Verification items for the finished model (mm, model axes). A direction names the side the tool comes from. Round coordinates to 2 decimals unless told otherwise and drop trailing zeros. Write each loop counter-clockwise with the first axis right and the second up, starting at its lowest first coordinate (ties: lowest second). Pieces come first, ordered by that corner, then holes. Notation, with made-up numbers: (85, 5) - (89, 5) arc R6 ccw to (89, 13) - close; hole circle Ø6 at (11, 30). An arc over 180 degrees is marked (long way). Write each question's results on one line, items separated by ' | '.
```python
from build123d import *

# Parameters (mm, degrees)
SKETCH1_R           = 18.5
BOSS_EXTRUDE1_DEPTH = 6
SKETCH3_R           = 2
CUT_EXTRUDE1_DEPTH  = 6
SKETCH7_R           = 3
BOSS_EXTRUDE4_DEPTH = 18
FILLET3_R           = 8
SKETCH8_R           = 4.5
CUT_EXTRUDE2_DEPTH  = 10


with BuildPart() as part:
    # Sketch1 → Boss-Extrude1 (new body)
    with BuildSketch(Plane.XY):
        Circle(SKETCH1_R)
    extrude(amount=BOSS_EXTRUDE1_DEPTH)

    # Sketch3 → Cut-Extrude1 (cut)
    with BuildSketch(Plane.XY.offset(6)):
        with Locations((-14, 0)):
            Circle(SKETCH3_R)
        with Locations((-7, 12.124355653)):
            Circle(SKETCH3_R)
        with Locations((7, 12.124355653)):
            Circle(SKETCH3_R)
        with Locations((14, 0)):
            Circle(SKETCH3_R)
        with Locations((7, -12.124355653)):
            Circle(SKETCH3_R)
        with Locations((-7, -12.124355653)):
            Circle(SKETCH3_R)
    extrude(amount=-CUT_EXTRUDE1_DEPTH, mode=Mode.SUBTRACT)

    # Sketch7 → Boss-Extrude4 (add)
    with BuildSketch(Plane.XY.offset(24)):
        Circle(SKETCH7_R)
    extrude(amount=-BOSS_EXTRUDE4_DEPTH)

    # Fillet3
    fillet3_edges = [part.edges().sort_by_distance(p)[0] for p in [
        (-3, 0, 6),
    ]]
    fillet(fillet3_edges, radius=FILLET3_R)

    # Sketch8 → Cut-Extrude2 (cut)
    with BuildSketch(Plane.XY.offset(6)):
        with Locations((-14, 0)):
            Circle(SKETCH8_R)
        with Locations((-7, 12.124355653)):
            Circle(SKETCH8_R)
        with Locations((7, 12.124355653)):
            Circle(SKETCH8_R)
        with Locations((14, 0)):
            Circle(SKETCH8_R)
        with Locations((7, -12.124355653)):
            Circle(SKETCH8_R)
        with Locations((-7, -12.124355653)):
            Circle(SKETCH8_R)
    extrude(amount=CUT_EXTRUDE2_DEPTH, mode=Mode.SUBTRACT)


solid = part.part
```
(1) Thickness scan on L1, parallel to X at y = 12, z = 2.5; L2, parallel to Y at x = -8.5, z = 5.5; L3, parallel to X at y = 11, z = 1.25. Record the ranges inside material, lowest first.
Answer:
L1: -14.08 to -9, -5 to 5, 9 to 14.08 | L2: -16.43 to -13.45, -10.8 to 10.8, 13.45 to 16.43 | L3: -14.87 to -8.65, -5.35 to 5.35, 8.65 to 14.87
(2) Set-up check for faces 1 (the cylindrical face through (-8.5, -10.8, 3)), 2 (the flat face through (8, -8, 6)): record each of +Z, -Z, +X, -X, +Y, -Y from which the full face is reachable in a straight line by a thin tool's end or side.
Answer:
face 1: +Z, -Z | face 2: +Z
(3) Section check C-C (x = -15). Record the cut outline in (y, z).
Answer:
outline: (-10.83, 0) - (-1.73, 0) - (-1.73, 6) - (-10.83, 6) - close; (1.73, 0) - (10.83, 0) - (10.83, 6) - (1.73, 6) - close
(4) Section check B-B (x = 0). Record the cut outline in (y, z).
Answer:
outline: (-18.5, 0) - (18.5, 0) - (18.5, 6) - (11, 6) arc R8 cw to (3, 14) - (3, 24) - (-3, 24) - (-3, 14) arc R8 cw to (-11, 6) - (-18.5, 6) - close
(5) Section check D-D (z = 11.5). Record the cut outline in (x, y), plus the area to 3 significant figures.
Answer:
outline: circle Ø6.8 at (0, 0) | area: 36.3 mm2
(6) Go/stop test with flat-tipped pins: pin 1 Ø4.5 at (x, y) = (-7, 12.12) entering from +Z; pin 2 Ø12 at (x, z) = (3, 15) entering from +Y; pin 3 Ø8 at (x, z) = (-10.5, 14) entering from +Y; pin 4 Ø12 at (y, z) = (0.5, 13.5) entering from -X. Record where each tip stops, or that it passes through.
Answer:
pin 1: z = 6 | pin 2: y = 4.38 | pin 3: through | pin 4: x = -6.32
(7) Section check A-A (y = 0). Record the cut outline in (x, z), plus the area to 3 significant figures.
Answer:
outline: (-18.5, 0) - (-16, 0) - (-16, 6) - (-18.5, 6) - close; (-12, 0) - (12, 0) - (12, 6) - (9.5, 6) - (9.5, 6.14) arc R8 cw to (3, 14) - (3, 24) - (-3, 24) - (-3, 14) arc R8 cw to (-9.5, 6.14) - (-9.5, 6) - (-12, 6) - close; (16, 0) - (18.5, 0) - (18.5, 6) - (16, 6) - close | area: 309 mm2
